Model file for the job. Use its own axes, mm. A direction names the side the tool comes from. Round coordinates to 2 decimals unless told otherwise and drop trailing zeros. Loops run counter-clockwise (first coordinate to the right, second up) from the corner with the lowest first, then second, coordinate; pieces in that order, holes last. Notation, with made-up numbers: M -32,-36.5 L -19,-36.5 A23 cw -19,-27.5 Z; hole C 7,-8 d5. An arc over 180 degrees is marked long. Answer in a Markdown table with one row per item.
from build123d import *

# Parameters (mm, degrees)
SKETCH1_W           = 18.8
SKETCH1_H           = 14
SKETCH1_W_2         = 16.5
SKETCH1_H_2         = 12
BOSS_EXTRUDE1_DEPTH = 7
SKETCH2_W           = 22.5
SKETCH2_H           = 18
SKETCH2_W_2         = 18.8
SKETCH2_H_2         = 14
SKETCH2_W_3         = 16.5
SKETCH2_H_3         = 12
BOSS_EXTRUDE2_DEPTH = 2
FILLET2_R           = 1
BOSS_EXTRUDE6_DEPTH = 16.8


with BuildPart() as part:
    # Sketch1 → Boss-Extrude1 (new body)
    with BuildSketch(Plane(origin=(0, 0, 0), x_dir=(1, 0, 0), z_dir=(0, 1, 0))):
        Rectangle(SKETCH1_W, SKETCH1_H)
        Rectangle(SKETCH1_W_2, SKETCH1_H_2, mode=Mode.SUBTRACT)
    extrude(amount=BOSS_EXTRUDE1_DEPTH)

    # Sketch2 → Boss-Extrude2 (add)
    # profile 1 of 2: a face of its own
    with BuildSketch(Plane(origin=(0, 0, 0), x_dir=(1, 0, 0), z_dir=(0, 1, 0))):
        Rectangle(SKETCH2_W, SKETCH2_H)
        Rectangle(SKETCH2_W_2, SKETCH2_H_2, mode=Mode.SUBTRACT)
    # profile 2 of 2: a face of its own
    with BuildSketch(Plane(origin=(0, 0, 0), x_dir=(1, 0, 0), z_dir=(0, 1, 0))):
        Rectangle(SKETCH2_W_2, SKETCH2_H_2)
        Rectangle(SKETCH2_W_3, SKETCH2_H_3, mode=Mode.SUBTRACT)
    extrude(amount=-BOSS_EXTRUDE2_DEPTH)

    # Fillet2
    fillet2_edges = [part.edges().sort_by_distance(p)[0] for p in [
        (8.25, 2.5, 6),
        (8.25, 2.5, -6),
        (-8.25, 2.5, -6),
        (-8.25, 2.5, 6),
        (11.25, -1, -9),
        (11.25, -1, 9),
        (-11.25, -1, 9),
        (-11.25, -1, -9),
        (9.4, 3.5, 7),
        (-9.4, 3.5, 7),
        (-9.4, 3.5, -7),
        (9.4, 3.5, -7),
    ]]
    fillet(fillet2_edges, radius=FILLET2_R)

    # Sketch7 → Boss-Extrude6 (add)
    with BuildSketch(Plane(origin=(-8.4, 0, 0), x_dir=(0, 0, -1), z_dir=(1, 0, 0))):
        with BuildLine():
            ThreePointArc((7, 3.2), (6.5, 2.7), (7, 2.2))
            Line((7, 2.2), (7, 3.2))
        make_face()
        with BuildLine():
            Line((7, 3.2), (7, 2.2))
            ThreePointArc((7, 2.2), (7.353553391, 2.346446609), (7.5, 2.7))
            ThreePointArc((7.5, 2.7), (7.353553391, 3.053553391), (7, 3.2))
        make_face()
        with BuildLine():
            ThreePointArc((-7, 3.2), (-7.5, 2.7), (-7, 2.2))
            Line((-7, 2.2), (-7, 3.2))
        make_face()
        with BuildLine():
            Line((-7, 3.2), (-7, 2.2))
            ThreePointArc((-7, 2.2), (-6.646446609, 2.346446609), (-6.5, 2.7))
            ThreePointArc((-6.5, 2.7), (-6.646446609, 3.053553391), (-7, 3.2))
        make_face()
    extrude(amount=BOSS_EXTRUDE6_DEPTH)


solid = part.part
1. Saw through at D-D (y = 5.75). Write the cut outline in (x, z).
Verdict:
| item | result |
|---|---|
| outline | M -9.4,-6 A1 ccw -8.4,-7 L 8.4,-7 A1 ccw 9.4,-6 L 9.4,6 A1 ccw 8.4,7 L -8.4,7 A1 ccw -9.4,6 Z; hole M -8.25,-5 A1 ccw -7.25,-6 L 7.25,-6 A1 ccw 8.25,-5 L 8.25,5 A1 ccw 7.25,6 L -7.25,6 A1 ccw -8.25,5 Z |
2. Pin check, flat tips, straight feed: pin 1 (1 mm diameter, centred on y = 1, z = -4.5, fed in from +X); pin 2 (2 mm diameter, centred on y = 2, z = -1, fed in from -X); pin 3 (2.5 mm diameter, centred on x = -1.5, y = 2, fed in from -Z); pin 4 (1.1 mm diameter, centred on x = 1.5, y = 0.5, fed in from +Z). Stop position of each tip, or through.
Verdict:
| item | result |
|---|---|
| pin 1 | stops at x = 9.4 |
| pin 2 | stops at x = -9.4 |
| pin 3 | stops at z = -7.5 |
| pin 4 | stops at z = 9 |
3. Saw through at C-C (z = 4). Write the cut outline in (x, y), and give its area (3 significant figures).
Verdict:
| item | result |
|---|---|
| outline | M -11.25,-2 L -8.25,-2 L -8.25,7 L -9.4,7 L -9.4,0 L -11.25,0 Z; M 8.25,-2 L 11.25,-2 L 11.25,0 L 9.4,0 L 9.4,7 L 8.25,7 Z |
| area | 28.1 mm² |
4. Saw through at A-A (x = -3.5). Write the cut outline in (y, z), and give its area (3 significant figures).
Verdict:
| item | result |
|---|---|
| outline | M -2,-9 L 0,-9 L 0,-7 L 2.2,-7 A0.5 ccw 3.2,-7 L 7,-7 L 7,-6 L -2,-6 Z; M -2,6 L 7,6 L 7,7 L 3.2,7 A0.5 ccw 2.2,7 L 0,7 L 0,9 L -2,9 Z |
| area | 26.8 mm² |
5. Tool access for faces 1 (the cylindrical face through (-9.099, 3.549, -6.715)), 2 (the flat face through (8.25, 3, 0)), 3 (the flat face through (-9.4, 3, 0)): list every direction of +Z, -Z, +X, -X, +Y, -Y with a clear straight run to the whole face (end or side of a thin tool).
Verdict:
| item | result |
|---|---|
| face 1 | -Z, -X, +Y |
| face 2 | +Y, -Y |
| face 3 | +Z, -Z, -X, +Y |
6. Saw through at B-B (y = -0.5). Write the cut outline in (x, z).
Verdict:
| item | result |
|---|---|
| outline | M -11.25,-8 A1 ccw -10.25,-9 L 10.25,-9 A1 ccw 11.25,-8 L 11.25,8 A1 ccw 10.25,9 L -10.25,9 A1 ccw -11.25,8 Z; hole M -8.25,-5 A1 ccw -7.25,-6 L 7.25,-6 A1 ccw 8.25,-5 L 8.25,5 A1 ccw 7.25,6 L -7.25,6 A1 ccw -8.25,5 Z |
7. Wall check: probe 1 along Z at (x, y) = (1.5, 0.5); probe 2 along X at (y, z) = (0.25, -3); probe 3 along X at (y, z) = (-1.25, 4). Give the ranges that are in metal, low to high.
Verdict:
| item | result |
|---|---|
| probe 1 | z = -7 to -6, 6 to 7 |
| probe 2 | x = -9.4 to -8.25, 8.25 to 9.4 |
| probe 3 | x = -11.25 to -8.25, 8.25 to 11.25 |
8. Mould opens along Z. For faces 4 (the flat face through (0, 3, -6)), 5 (the cylindrical face through (-0.1, 2.7, 7.5)), 6 (the flat face through (0, -2, -8)) say: +Z half, -Z half, draft (parallel to the pull), parting line (faces both ways), or undercut.
Verdict:
| item | result |
|---|---|
| face 4 | undercut |
| face 5 | +Z half |
| face 6 | draft |
